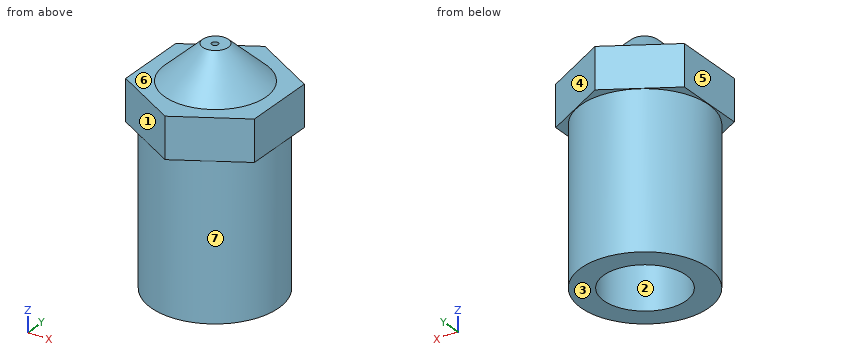
Autodesk Inventor part; units mm, degrees
ref_plane "Work Plane1" through (0, -2.3094, 9.54) normal (1, 0, 0) x (0, 0, -1)
ref_plane "YZ Plane" through (0, 0, 0) normal (1, 0, 0) x (0, 1, 0)
ref_plane "XZ Plane" through (0, 0, 0) normal (0, 1, 0) x (-1, 0, 0)
sketch "Sketch1" plane through (0, 0, 0) normal (0, 0, 1) x (1, 0, 0)
  circle A0 centre (0, 0) radius 3.965
  dimension "d0" = 7.93
extrude "Extrusion1" add sketch "Sketch1" along normal blind 9.54
sketch "Sketch2" plane through (0, 0, 9.54) normal (0, 0, 1) x (1, 0, 0)
  circle A0 centre (0, 0) radius 3.965
  line L0 (0, 4.6188) -> (4, 2.3094)
  line L1 (4, 2.3094) -> (4, -2.3094)
  line L2 (4, -2.3094) -> (0, -4.6188)
  line L3 (0, -4.6188) -> (-4, -2.3094)
  line L4 (-4, -2.3094) -> (-4, 2.3094)
  line L5 (-4, 2.3094) -> (0, 4.6188)
  dimension "d4" = 8
extrude "Extrusion2" add sketch "Sketch2" along normal blind 2.54 contours A0 | L0 L1 L2 L3 L4 L5
ref_plane "Work Plane1" through (0, -2.3094, 9.54) normal (1, 0, 0) x (0, 0, -1)
sketch "Sketch3" plane through (0, -2.3094, 9.54) normal (1, 0, 0) x (0, 0, -1)
  line L0 (-2.54, 2.3576) -> (-4.74, 2.3576)
  line L1 (-4.74, 3.1576) -> (-2.54, 5.5076)
  line L2 (-4.74, 3.1576) -> (-4.74, 2.3576)
  line L3 (-2.54, 0) -> (-2.54, 4.6188)
  line L4 (9.54, 2.3094) -> (2.1715, 2.3094)
  line L5 (-2.54, 4.6188) -> (-2.54, 6.9282)
  line L6 (-2.54, 5.5076) -> (-2.54, 2.3576)
  point P0 (-2.54, 2.3094)
  dimension "d7" = 3.15
  dimension "d9" = 2.2
  dimension "d10" = 0.8
revolve "Revolution1" add sketch "Sketch3" angle 360 about axis through (0, 0.0482, 12.08) along (0, 0, 1)
sketch "Sketch4" plane through (0, 0.0482, 14.28) normal (0, 0, 1) x (1, 0, 0)
  circle A0 centre (0, -0.0482) radius 0.2
  dimension "d12" = 0.4
extrude "Extrusion3" cut sketch "Sketch4" against normal through all
sketch "Sketch5" plane through (0, 0, 0) normal (0, 0, -1) x (-1, 0, 0)
  circle A0 centre (0, 0) radius 0.2
  circle A1 centre (0, 0) radius 2.55
  point P0 (0, 0)
  dimension "d15" = 5.1
extrude "Extrusion4" cut sketch "Sketch5" against normal blind 9.17 contours A0 | A1
thread "Thread1"
properties part number "nozzel" material "Brass, Soft Yellow"
Source: CAD feature listing. Evaluate the final solid. Frame: model axes, mm. Face numbers are marked on the shaded views. A direction names the side the tool comes from. Round coordinates to 2 decimals unless told otherwise and drop trailing zeros. Loops run counter-clockwise (first coordinate to the right, second up) from the corner with the lowest first, then second, coordinate; pieces in that order, holes last. Notation, with made-up numbers: (-7.75, -18.5) - (3.25, -18.5) arc R17 ccw to (3.25, 14.5) - close; hole circle Ø9 at (-23.75, 50.25). An arc over 180 degrees is marked (long way). Write item = value, one per line. Start each with the question number.
(1) Ray query, line 1 along Y through (x, z) = (0, 4.25) (3 decimals); line 2 along Z through (x, y) = (-1.5, -3.5); line 3 along X through (y, z) = (-0.5, 0.5). Return the intervals inside material, ascending. Write a range as from..to.
(2) Set-up query: the marked faces 5, 6 and 7. Return all of +Z, -Z, +X, -X, +Y, -Y with unobstructed straight access to the full face (end or side cutting, diameter ignored); none if empty.
(3) Section query C-C, the plane z = 13. Output: boundary loops of the cut face in (x, y), plus the area to 3 significant figures.
(4) Section query A-A, the plane z = 10. Output: boundary loops of the cut face in (x, y).
(5) Pin query (flat end, axial travel): pin 1 (5 mm diameter, centred on y = -3, z = 4.5, fed in from +X); pin 2 (4 mm diameter, centred on x = 1.5, y = 2, fed in from -Z); pin 3 (2 mm diameter, centred on x = 1, z = 8, fed in from +Y) (3 decimals); pin 4 (1 mm diameter, centred on x = 2.5, z = 5, fed in from -Y). Return the tip coordinate at first contact, or that it passes through.
(6) Section query B-B, the plane z = 4.5. Output: boundary loops of the cut face in (x, y) (3 decimals), plus the area to 3 significant figures.
(7) Pull-direction query (X, two-part tool) for the marked faces 1, 2, 3 and 4; classes: +X half, -X half, draft (parallel to the pull), parting line (faces both ways), or undercut.
Conclusion:
q1.line_1 = -3.965..-2.55, 2.55..3.965
q1.line_2 = 0..12.08
q1.line_3 = -3.93..-2.5, 2.5..3.93
q2.face_5 = +Z, -Z, -X, +Y, -Y
q2.face_6 = +Z
q2.face_7 = -Z
q3.outline = circle Ø4.33 at (0, 0.05); hole circle Ø0.4 at (0, 0)
q3.area = 14.6 mm2
q4.outline = (-4, -2.31) - (0, -4.62) - (4, -2.31) - (4, 2.31) - (0, 4.62) - (-4, 2.31) - close; hole circle Ø0.4 at (0, 0)
q5.pin_1 = 3.93
q5.pin_2 = 0
q5.pin_3 = 3.965
q5.pin_4 = -3.42
q6.outline = circle Ø7.93 at (0, 0); hole circle Ø5.1 at (0, 0)
q6.area = 29.0 mm2
q7.face_1 = -X half
q7.face_2 = undercut
q7.face_3 = draft
q7.face_4 = +X half
